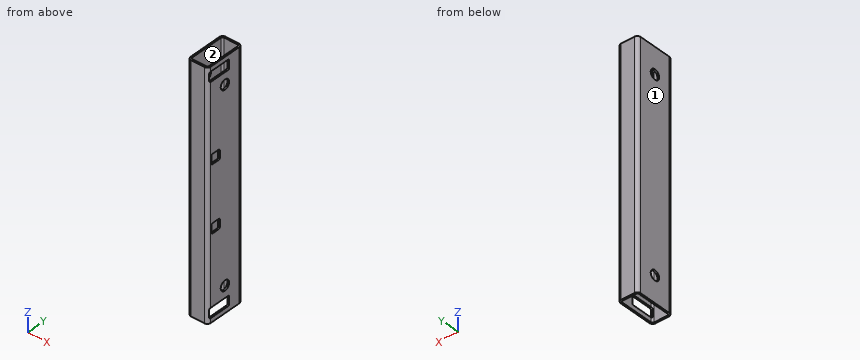
```python
from build123d import *

# Parameters (mm, degrees)
BOSS_EXTRUDE1_DEPTH                       = 925
CUT_EXTRUDE1_DEPTH                        = 30
FOR_MACH_SHOP_CONFIRM_W_PROGRAMMING_REACH = 951.777
SKETCH5_R                                 = 37.5
CUT_EXTRUDE3_DEPTH                        = 950.777089767


with BuildPart() as part:
    # Sketch1 → Boss-Extrude1 (new, symmetric)
    with BuildSketch(Plane.XY):
        with BuildLine():
            Line((-50.8, -152.4), (50.8, -152.4))
            ThreePointArc((50.8, -152.4), (68.760512242, -144.960512242), (76.2, -127))
            Line((76.2, -127), (76.2, 127))
            ThreePointArc((76.2, 127), (68.760512242, 144.960512242), (50.8, 152.4))
            Line((50.8, 152.4), (-50.8, 152.4))
            ThreePointArc((-50.8, 152.4), (-68.760512242, 144.960512242), (-76.2, 127))
            Line((-76.2, 127), (-76.2, -127))
            ThreePointArc((-76.2, -127), (-68.760512242, -144.960512242), (-50.8, -152.4))
        make_face()
        with BuildLine():
            Line((-50.8, -139.7), (50.8, -139.7))
            ThreePointArc((50.8, -139.7), (59.780256121, -135.980256121), (63.5, -127))
            Line((63.5, -127), (63.5, 127))
            ThreePointArc((63.5, 127), (59.780256121, 135.980256121), (50.8, 139.7))
            Line((50.8, 139.7), (-50.8, 139.7))
            ThreePointArc((-50.8, 139.7), (-59.780256121, 135.980256121), (-63.5, 127))
            Line((-63.5, 127), (-63.5, -127))
            ThreePointArc((-63.5, -127), (-59.780256121, -135.980256121), (-50.8, -139.7))
        make_face(mode=Mode.SUBTRACT)
    extrude(amount=BOSS_EXTRUDE1_DEPTH, both=True)

    # Sketch2 → Cut-Extrude1 (cut)
    with BuildSketch(Plane(origin=(76.2, 0, 0), x_dir=(0, 0, -1), z_dir=(1, 0, 0))):
        with BuildLine():
            Line((-880, 37.6), (-825, 37.6))
            ThreePointArc((-825, 37.6), (-817.928932188, 34.671067812), (-815, 27.6))
            Line((-815, 27.6), (-815, -127.4))
            ThreePointArc((-815, -127.4), (-817.928932188, -134.471067812), (-825, -137.4))
            Line((-825, -137.4), (-880, -137.4))
            ThreePointArc((-880, -137.4), (-887.071067812, -134.471067812), (-890, -127.4))
            Line((-890, -127.4), (-890, 27.6))
            ThreePointArc((-890, 27.6), (-887.071067812, 34.671067812), (-880, 37.6))
        make_face()
        with BuildLine():
            Line((825, 37.6), (880, 37.6))
            ThreePointArc((880, 37.6), (887.071067812, 34.671067812), (890, 27.6))
            Line((890, 27.6), (890, -127.4))
            ThreePointArc((890, -127.4), (887.071067812, -134.471067812), (880, -137.4))
            Line((880, -137.4), (825, -137.4))
            ThreePointArc((825, -137.4), (817.928932188, -134.471067812), (815, -127.4))
            Line((815, -127.4), (815, 27.6))
            ThreePointArc((815, 27.6), (817.928932188, 34.671067812), (825, 37.6))
        make_face()
    extrude(amount=-CUT_EXTRUDE1_DEPTH, mode=Mode.SUBTRACT)

    # Sketch3 → for mach shop confirm w/ programming (cut, up to next)
    with BuildSketch(Plane(origin=(76.2, 0, 0), x_dir=(0, 0, -1), z_dir=(1, 0, 0)), mode=Mode.PRIVATE) as for_mach_shop_confirm_w_programming_sk1:
        with BuildLine():
            Line((-277.5, -45.65), (-222.5, -45.65))
            ThreePointArc((-222.5, -45.65), (-215.428932188, -48.578932188), (-212.5, -55.65))
            Line((-212.5, -55.65), (-212.5, -110.65))
            ThreePointArc((-212.5, -110.65), (-215.428932188, -117.721067812), (-222.5, -120.65))
            Line((-222.5, -120.65), (-277.5, -120.65))
            ThreePointArc((-277.5, -120.65), (-284.571067812, -117.721067812), (-287.5, -110.65))
            Line((-287.5, -110.65), (-287.5, -55.65))
            ThreePointArc((-287.5, -55.65), (-284.571067812, -48.578932188), (-277.5, -45.65))
        make_face()
    for_mach_shop_confirm_w_programming_tool1 = extrude(for_mach_shop_confirm_w_programming_sk1.sketch, amount=-FOR_MACH_SHOP_CONFIRM_W_PROGRAMMING_REACH, mode=Mode.PRIVATE) & part.part
    # Sketch3 → for mach shop confirm w/ programming (cut, up to next)
    with BuildSketch(Plane(origin=(76.2, 0, 0), x_dir=(0, 0, -1), z_dir=(1, 0, 0)), mode=Mode.PRIVATE) as for_mach_shop_confirm_w_programming_sk2:
        with BuildLine():
            Line((222.5, -45.65), (277.5, -45.65))
            ThreePointArc((277.5, -45.65), (284.571067812, -48.578932188), (287.5, -55.65))
            Line((287.5, -55.65), (287.5, -110.65))
            ThreePointArc((287.5, -110.65), (284.571067812, -117.721067812), (277.5, -120.65))
            Line((277.5, -120.65), (222.5, -120.65))
            ThreePointArc((222.5, -120.65), (215.428932188, -117.721067812), (212.5, -110.65))
            Line((212.5, -110.65), (212.5, -55.65))
            ThreePointArc((212.5, -55.65), (215.428932188, -48.578932188), (222.5, -45.65))
        make_face()
    for_mach_shop_confirm_w_programming_tool2 = extrude(for_mach_shop_confirm_w_programming_sk2.sketch, amount=-FOR_MACH_SHOP_CONFIRM_W_PROGRAMMING_REACH, mode=Mode.PRIVATE) & part.part
    add(for_mach_shop_confirm_w_programming_tool1.solids().sort_by_distance((76.2, -83.15, 250))[0], mode=Mode.SUBTRACT)
    add(for_mach_shop_confirm_w_programming_tool2.solids().sort_by_distance((76.2, -83.15, -250))[0], mode=Mode.SUBTRACT)

    # Sketch5 → Cut-Extrude3 (cut, through all)
    with BuildSketch(Plane.ZY.offset(76.2)):
        with Locations((725, 0)):
            Circle(SKETCH5_R)
        with Locations((-725, 0)):
            Circle(SKETCH5_R)
    extrude(amount=-CUT_EXTRUDE3_DEPTH, mode=Mode.SUBTRACT)


solid = part.part
```
The model under review builds one solid part; all positions refer to its coordinate system, in mm. Face numbers are marked on the shaded views. Round coordinates to 2 decimals unless told otherwise and drop trailing zeros. Write each loop counter-clockwise with the first axis right and the second up, starting at its lowest first coordinate (ties: lowest second). Pieces come first, ordered by that corner, then holes.
(1) We need section D-D on y = 80. Give the boundary of the cut face in (x, z), and give its area (3 significant figures).
(2) We need section A-A on z = 725. Give the boundary of the cut face in (x, y).
(3) Wall thickness on L1, parallel to X at y = 95.5, z = -498; L2, parallel to Y at x = -47, z = 430; L3, parallel to Z at x = 65.5, y = 15: over which ranges is each line inside the solid? List them lowest first.
(4) We need section C-C on y = 0. Give the number of separate pieces and of enclosed holes in the cut face, and give its area (3 significant figures).
(5) Insertion check: pin 1 (4 mm diameter, centred on x = 68, z = 260, fed in from +Y); pin 2 (10 mm diameter, centred on x = 69, z = 859, fed in from -Y); pin 3 (17.5 mm diameter, centred on x = 64.5, z = 841.5, fed in from +Y). Each pin has a flat end and moves straight along its axis. Give the tip position at first contact, or say it passes through.
(6) We need section B-B on x = 26.5. Give the boundary of the cut face in (y, z), and give its area (3 significant figures).
(7) Mouldability with a two-part tool opening along Y and no side actions: class the marked faces 1 and 2 as +Y half, -Y half, draft (parallel to the pull), parting line (faces both ways), or undercut.
Findings below:
1. outline: (-76.2, -925) - (-63.5, -925) - (-63.5, 925) - (-76.2, 925) - close; (63.5, -925) - (76.2, -925) - (76.2, 925) - (63.5, 925) - close
1. area: 47,000 mm2
2. outline: (-76.2, -127) arc R25.4 ccw to (-50.8, -152.4) - (50.8, -152.4) arc R25.4 ccw to (76.2, -127) - (76.2, -37.5) - (63.5, -37.5) - (63.5, -127) arc R12.7 cw to (50.8, -139.7) - (-50.8, -139.7) arc R12.7 cw to (-63.5, -127) - (-63.5, -37.5) - (-76.2, -37.5) - close; (-76.2, 37.5) - (-63.5, 37.5) - (-63.5, 127) arc R12.7 cw to (-50.8, 139.7) - (50.8, 139.7) arc R12.7 cw to (63.5, 127) - (63.5, 37.5) - (76.2, 37.5) - (76.2, 127) arc R25.4 ccw to (50.8, 152.4) - (-50.8, 152.4) arc R25.4 ccw to (-76.2, 127) - close
3. L1: x = -76.2 to -63.5, 63.5 to 76.2
3. L2: y = -152.4 to -139.7, 139.7 to 152.4
3. L3: z = -925 to -890, -815 to -759.37, -690.63 to 690.63, 759.37 to 815, 890 to 925
4. separate pieces: 8
4. enclosed holes: 0
4. area: 41,300 mm2
5. pin 1: stops at y = 147.35
5. pin 2: stops at y = -148.7
5. pin 3: stops at y = 151.91
6. outline: (-152.4, -925) - (-139.7, -925) - (-139.7, 925) - (-152.4, 925) - close; (139.7, -925) - (152.4, -925) - (152.4, 925) - (139.7, 925) - close
6. area: 47,000 mm2
7. face 1: draft
7. face 2: undercut
